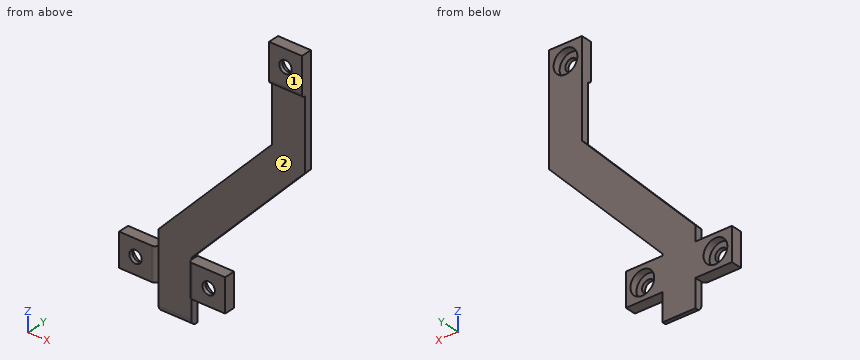
Autodesk Inventor part; units mm, degrees
ref_plane "YZ Plane" through (0, 0, 0) normal (1, 0, 0) x (0, 1, 0)
ref_plane "XZ Plane" through (0, 0, 0) normal (0, 1, 0) x (-1, 0, 0)
ref_plane "XY Plane" through (0, 0, 0) normal (0, 0, 1) x (1, 0, 0)
sketch "Sketch1" plane through (0, 0, 0) normal (0, 1, 0) x (-1, 0, 0)
  line L0 (0, 0) -> (-10, 0)
  line L1 (-10, 0) -> (-10, -51)
  line L2 (-10, -51) -> (0, -51)
  line L3 (0, -51) -> (0, 0)
  line L4 (0, 0) -> (-41, 0)
  line L5 (-41, 0) -> (-41, -10)
  line L6 (-41, -10) -> (0, -10)
  line L7 (0, -10) -> (0, 0)
  line L8 (-41, -10) -> (-31, -10)
  line L9 (-31, -10) -> (-31, 30)
  line L10 (-31, 30) -> (-41, 30)
  line L11 (-41, 30) -> (-41, -10)
  line L12 (-10, -51) -> (-10, -43)
  line L13 (-10, -43) -> (-20, -43)
  line L14 (-20, -43) -> (10, -43)
  line L15 (10, -43) -> (10, -33)
  line L16 (10, -33) -> (-20, -33)
  line L17 (-20, -33) -> (-20, -43)
  point P0 (0, -43)
  point P1 (0, -33)
  point P2 (-31, 0)
  point P3 (-10, -10)
  point P4 (-10, -33)
  dimension "d0" = 10
  dimension "d1" = 51
  dimension "d2" = 41
  dimension "d3" = 10
  dimension "d4" = 10
  dimension "d5" = 40
  dimension "d6" = 8
  dimension "d7" = 10
  dimension "d8" = 30
  dimension "d9" = 10
extrude "Extrusion1" add sketch "Sketch1" along normal blind 3
sketch "Sketch2" plane through (0, 3, 0) normal (0, 1, 0) x (1, 0, 0)
  line L0 (-10, 33) -> (0, 33)
  line L1 (0, 33) -> (0, 38)
  line L2 (0, 38) -> (-5, 38)
  circle A0 centre (-5, 38) radius 3.25
  line L3 (0, 38) -> (15, 38)
  circle A1 centre (15, 38) radius 3.25
  line L4 (41, -30) -> (41, 10)
  line L5 (41, -30) -> (41, -25)
  line L6 (41, -25) -> (41, -30)
  line L7 (41, -25) -> (36, -25)
  circle A2 centre (36, -25) radius 3.25
  circle A3 centre (-5, 38) radius 1.7
  circle A4 centre (15, 38) radius 1.7
  circle A5 centre (36, -25) radius 1.7
  point P0 (0, 0)
  dimension "d12" = 5
  dimension "d13" = 5
  dimension "d14" = 6.5
  dimension "d15" = 15
  dimension "d16" = 6.5
  dimension "d17" = 5
  dimension "d18" = 5
  dimension "d19" = 5
  dimension "d20" = 6.5
  dimension "d23" = 3.4
  dimension "d24" = 3.4
  dimension "d25" = 3.4
extrude "Extrusion3" cut sketch "Sketch2" against normal blind 2
extrude "Extrusion4" cut sketch "Sketch2" against normal blind 4 contours A3 | A4 | A5
sketch "Sketch3" plane through (0, 3, 0) normal (0, 1, 0) x (1, 0, 0)
  line L0 (0, 0) -> (0, 0.5)
  line L1 (0, 33) -> (0, 0)
  line L2 (0, 0.5) -> (31, 0.5)
  line L3 (31, 0.5) -> (31.5, 0.5)
  line L4 (31.5, 0.5) -> (31.5, -21.5)
  line L5 (31.5, -21.5) -> (40.5, -21.5)
  line L6 (31, -30) -> (41, -30)
  line L7 (40.5, -21.5) -> (40.5, 9.5)
  line L8 (41, -30) -> (41, 10)
  line L9 (40.5, 9.5) -> (9.5, 9.5)
  line L10 (9.5, 9.5) -> (9.5, 33.5)
  line L11 (9.5, 33.5) -> (19.5, 33.5)
  line L12 (20, 33) -> (20, 43)
  line L13 (19.5, 33.5) -> (19.5, 42.5)
  line L14 (19.5, 42.5) -> (9.5, 42.5)
  line L15 (9.5, 42.5) -> (9.5, 51)
  line L16 (10, 51) -> (0, 51)
  line L17 (10, 43) -> (10, 51)
  line L18 (9.5, 51) -> (10, 51)
  line L19 (10, 51) -> (10, 43)
  line L20 (20, 43) -> (10, 43)
  line L21 (20, 43) -> (10, 43)
  line L22 (10, 33) -> (20, 33)
  line L23 (20, 43) -> (20, 33)
  line L24 (20, 33) -> (10, 33)
  line L25 (10, 33) -> (10, 10)
  line L26 (41, 10) -> (10, 10)
  line L27 (10, 10) -> (41, 10)
  line L28 (41, 10) -> (41, -30)
  line L29 (31, 0) -> (31, -30)
  line L30 (41, -30) -> (31, -30)
  line L31 (31, -30) -> (31, 0)
  line L32 (31, 0) -> (0, 0)
  line L33 (0, 0.5) -> (0.5, 0.5)
  line L34 (0.5, 0.5) -> (0.5, 33.5)
  line L35 (9.5, 11.7035) -> (0.5, 11.7035)
  line L36 (5, 11.7035) -> (5, 17)
  line L37 (0.5, 9.5) -> (0.5, 33.5)
  line L38 (0.5, 33.5) -> (-9.5, 33.5)
  line L39 (-10, 33) -> (-10, 43)
  line L40 (-9.5, 33.5) -> (-9.5, 42.5)
  line L41 (-9.5, 42.5) -> (0.5, 42.5)
  line L42 (0.5, 42.5) -> (0.5, 51)
  line L43 (0, 51) -> (10, 51)
  line L44 (0, 43) -> (0, 51)
  line L45 (0.5, 51) -> (0, 51)
  line L46 (0, 51) -> (0, 43)
  line L47 (-10, 43) -> (0, 43)
  line L48 (-10, 43) -> (0, 43)
  line L49 (0, 33) -> (-10, 33)
  line L50 (-10, 43) -> (-10, 33)
  line L51 (-10, 33) -> (0, 33)
  line L52 (0, 33) -> (0, 10)
  line L53 (0, 0) -> (0.5, 0)
  line L54 (0.5, 0) -> (0.5, 33.5)
  line L55 (0.5, 33.5) -> (0, 33.5)
  line L56 (0, 33.5) -> (0, 0)
  dimension "d30" = 0.5
  dimension "d31" = 31
  dimension "d32" = 90
  dimension "d33" = 0.5
  dimension "d34" = 22
  dimension "d35" = 9
  dimension "d36" = 90
  dimension "d37" = 31
  dimension "d38" = 90
  dimension "d39" = 31
  dimension "d40" = 24
  dimension "d41" = 10
  dimension "d42" = 9
  dimension "d43" = 0.5
extrude "Extrusion5" cut sketch "Sketch3" against normal blind 4 contours L0 L2 L54 L32 | L1 L56 L38 L34 L2 | L54 L2 L3 L4 L5 L7 L9 L10 L11 L13 L14 L15 L16 L17 L20 L12 L22 L25 L26 L8 L6 L29 L32 | L49 L39 L47 L44 L16 L42 L41 L40 L38 L56
sketch "Sketch4" plane through (0, 3, 0) normal (0, 1, 0) x (1, 0, 0)
  line L0 (40.5, 9.5) -> (40.5, 38.6053)
  line L1 (9.5, 33.5) -> (46.5578, 33.5)
  line L2 (40.5, 33.5) -> (40.5, 0.5)
  line L3 (40.5, 9.5) -> (40.5, -21.5)
  line L4 (9.5, 9.5) -> (9.5, 33.5)
  line L5 (40.5, 0) -> (9.5, 33)
  line L6 (40.5, 0) -> (33.9404, -6.1621)
  line L7 (33.9404, -6.1621) -> (-17.219, 48.2979)
  line L8 (0.5, 33.5) -> (0.5, 0.5)
  line L9 (0.5, 33) -> (0.5, 28.5562)
  line L10 (19.5, 33.5) -> (9.5, 33.5)
  line L11 (9.5, 33) -> (0.5, 33)
  line L12 (9.5, 33.5) -> (9.5, 33)
  line L13 (9.5, 33.5) -> (9.5, 9.5)
  point P0 (0, 0)
  point P1 (0.5, 29.4357)
  point P2 (0.5, 33)
  dimension "d49" = 33
  dimension "d50" = 9
  dimension "d55" = 0.5
sketch "Sketch5" plane through (0, 3, 0) normal (0, 1, 0) x (1, 0, 0)
  line L0 (0.5, 33.5) -> (31.5, 33.5)
  line L1 (31.5, 33.5) -> (31.5, 9.5)
  line L2 (31.5, 0.5) -> (0.5, 0.5)
  line L3 (0.5, 0.5) -> (0.5, 33.5)
  line L4 (9.5, 9.5) -> (40.5, 9.5)
  line L5 (31.5, 0.5) -> (40.5, 0.5)
  line L6 (40.5, 0.5) -> (40.5, 9.5)
  line L7 (40.5, 9.5) -> (31.5, 9.5)
  point P0 (0, 0)
extrude "Extrusion6" cut sketch "Sketch5" against normal blind 4
extrude "Extrusion7" add sketch "Sketch4" against normal blind 3 contours L6 L7 L4 L5 | L4 L7 L8 L11
sketch "Sketch6" plane through (0, 3, 0) normal (0, 1, 0) x (1, 0, 0)
  line L0 (40.0303, 0.5) -> (9.5, 33)
  line L1 (33.4215, 7.5352) -> (47.7617, -7.7302)
  line L2 (47.7617, -7.7302) -> (49.311, 2.3426)
  line L3 (49.311, 2.3426) -> (33.4215, 7.5352)
  line L4 (9.5, 33) -> (0.5, 33)
  line L5 (-9.5, 33.5) -> (19.5, 33.5)
  line L6 (0.5, 33) -> (9.5, 33)
  line L7 (9.5, 33) -> (9.5, 33.5)
  line L8 (9.5, 33.5) -> (0.5, 33.5)
  line L9 (0.5, 33.5) -> (0.5, 33)
  point P0 (0, 0)
extrude "Extrusion8" add sketch "Sketch6" against normal blind 3 contours L4 L9 L5 L7
sketch "Sketch7" plane through (0, 3, 0) normal (0, 1, 0) x (1, 0, 0)
  line L0 (9.5, 33) -> (40.0303, 0.5)
  line L1 (37.6071, 3.0795) -> (42.3492, -1.9686)
  line L2 (42.3492, -1.9686) -> (43.0836, 1.6709)
  line L3 (43.0836, 1.6709) -> (37.6071, 3.0795)
  point P0 (0, 0)
  point P1 (40.0303, 0.5)
extrude "Extrusion9" cut sketch "Sketch7" against normal blind 3
sketch "Sketch10" plane through (0, 3, 0) normal (0, 1, 0) x (1, 0, 0)
  line L0 (40.5, -21.5) -> (31.5, -21.5)
  line L1 (31.5, -21.5) -> (31.5, -29.5)
  line L2 (31.5, -29.5) -> (40.5, -29.5)
  line L3 (40.5, -29.5) -> (40.5, -21.5)
  point P0 (0, 0)
  dimension "d60" = 9
  dimension "d61" = 8
extrude "Extrusion10" add sketch "Sketch10" against normal blind 3
sketch "Sketch11" plane through (0, 3, 0) normal (0, 1, 0) x (1, 0, 0)
  line L0 (31.5, -29.5) -> (40.5, -29.5)
  line L1 (36, -29.5) -> (36, -25)
  circle A0 centre (36, -25) radius 1.7
  point P0 (0, 0)
  dimension "d64" = 4.5
  dimension "d65" = 3.4
extrude "Extrusion11" cut sketch "Sketch11" against normal blind 3
sketch "Sketch12" plane through (0, 3, 0) normal (0, 1, 0) x (1, 0, 0)
  circle A0 centre (36, -25) radius 1.7
  circle A1 centre (36, -25) radius 3.25
  point P0 (0, 0)
  dimension "d68" = 6.5
extrude "Extrusion12" cut sketch "Sketch12" against normal blind 2
sketch "Sketch13" plane through (0, 3, 0) normal (0, 1, 0) x (1, 0, 0)
  line L0 (9.5, 51) -> (9.5, 42.5)
  line L1 (0.5, 42.5) -> (0.5, 51)
  line L2 (9.5, 51) -> (0.5, 51)
  line L3 (0.5, 51) -> (0.5, 48.5)
  line L4 (0.5, 48.5) -> (9.5, 48.5)
  line L5 (9.5, 48.5) -> (9.5, 51)
  point P0 (0, 0)
  point P1 (9.5, 48.5)
  dimension "d71" = 2.5
extrude "Extrusion13" cut sketch "Sketch13" against normal blind 3
sketch "Sketch14" plane through (0, 0, 0) normal (0, -1, 0) x (1, 0, 0)
  line L0 (9.5, -48.5) -> (0.5, -48.5)
  line L1 (9.5, -48.5) -> (0.5, -48.5)
  line L2 (0.5, -48.5) -> (0.5, -29.4357)
  line L3 (0.5, -29.4357) -> (9.5, -29.4357)
  line L4 (9.5, -29.4357) -> (9.5, -48.5)
  line L5 (-9.5, -33.5) -> (0.5, -33.5)
  line L6 (40.5, 29.5) -> (40.5, 0)
  line L7 (0.5, -33.5) -> (40.5, -33.5)
  line L8 (40.5, -33.5) -> (40.5, 19)
  line L9 (40.5, 19) -> (0.5, 19)
  line L10 (0.5, 19) -> (0.5, -33.5)
  point P0 (0, 0)
  point P1 (9.5, -33.5)
  point P2 (40.5, 0)
  dimension "d76" = 52.5
extrude "Extrusion14" cut sketch "Sketch14" against normal blind 1
fillet "Fillet4" radius 1 3 edges at (0.5, 0, -38) (9.5, 0, -38) (36, 0, 19)
sketch "Sketch15" plane through (0, 1, 0) normal (0, -1, 0) x (1, 0, 0)
  line L0 (9.5, -42.5) -> (9.5, -48.5)
  line L1 (9.5, -48.5) -> (0.5, -48.5)
  line L2 (0.5, -48.5) -> (0.5, -50)
  line L3 (0.5, -50) -> (9.5, -50)
  line L4 (9.5, -50) -> (9.5, -48.5)
  point P0 (0, 0)
  dimension "d81" = 9
  dimension "d82" = 1.5
extrude "Extrusion15" add sketch "Sketch15" against normal blind 2
fillet "Fillet6" radius 1.5 1 edges at (5, 1, -50)
properties part number "Cover_bottom_raceway_cover"
Work out the finished part from the listing and answer in its coordinate system (mm). Face numbers are marked on the shaded views. A direction names the side the tool comes from. Coordinates: 2 decimals unless noted, no trailing zeros. Loops run counter-clockwise (first coordinate to the right, second up) from the corner with the lowest first, then second, coordinate; pieces in that order, holes last. Notation, with made-up numbers: (19, 69) -> (60, 69) arc R9 cw to (60, 75) -> close; hole circle Ø6 at (73, 13.25). An arc over 180 degrees is marked (long way). Write each question's results on one line, items separated by ' | '. Start each with the question number.
1) Find section A-A on z = -38. Count the separate pieces of the cut face and the enclosed holes in it, then the cut area to 3 significant figures.
2) Find section D-D on x = 15. Determine the outline of the cut face in (y, z), then the cut area to 3 significant figures.
3) Find section B-B on x = -5. Determine the outline of the cut face in (y, z), then the cut area to 3 significant figures.
4) Consider line 1 along X through (y, z) = (0.2, 25); line 2 along X through (y, z) = (0.5, -38); line 3 along Z through (x, y) = (15, 1.6). Determine where each line is inside the solid, lowest interval first.
5) For the marked faces 1 and 2, determine the directions among +Z, -Z, +X, -X, +Y, -Y from which every point of the face is accessible in a straight line to the end or side of a thin tool.
6) Find section C-C on y = 0.5. Determine the outline of the cut face in (x, z), then the cut area to 3 significant figures.
7) Flat-ended cylindrical pins translate along their axes: P1, Ø3, axis at x = 11.5, z = -20.5, coming from the -Y side; P2, Ø2.5, axis at x = 36, z = 25, coming from the -Y side; P3, Ø0.9, axis at x = 16.5, y = 1.5, coming from the +Z side; P4, Ø1.6, axis at y = 2, z = -44.5, coming from the +X side. Find the tip coordinate at first contact, or state that the pin passes through.
Response values:
1) separate pieces: 3 | enclosed holes: 0 | area: 44.8 mm^2
2) outline: (0, -42.5) -> (3, -42.5) -> (3, -41.25) -> (1, -41.25) -> (1, -39.7) -> (0, -39.7) -> close; (0, -36.3) -> (1, -36.3) -> (1, -34.75) -> (3, -34.75) -> (3, -33.5) -> (0, -33.5) -> close; (1, -27.15) -> (3, -27.15) -> (3, -14) -> (1, -14) -> close | area: 36.9 mm^2
3) outline: (0, -42.5) -> (3, -42.5) -> (3, -41.25) -> (1, -41.25) -> (1, -39.7) -> (0, -39.7) -> close; (0, -36.3) -> (1, -36.3) -> (1, -34.75) -> (3, -34.75) -> (3, -33.5) -> (0, -33.5) -> close | area: 10.6 mm^2
4) line 1: x = 31.5 to 34.3, 37.7 to 40.5 | line 2: x = -9.5 to -6.7, -3.3 to 0.37, 9.63 to 13.3, 16.7 to 19.5 | line 3: z = -42.5 to -41.25, -34.75 to -33.5, -27.15 to -14
5) face 1: +Z, -Z, +X, -X, -Y | face 2: -Y
6) outline: (-9.5, -42.5) -> (0.37, -42.5) -> (0.37, -33.5) -> (-9.5, -33.5) -> close; (9.63, -42.5) -> (19.5, -42.5) -> (19.5, -33.5) -> (9.63, -33.5) -> close; (31.5, 19.13) -> (40.5, 19.13) -> (40.5, 29.5) -> (31.5, 29.5) -> close; hole circle Ø3.4 at (-5, -38); hole circle Ø3.4 at (15, -38); hole circle Ø3.4 at (36, 25) | area: 244 mm^2
7) P1: stops at y = 1 | P2: passes through | P3: stops at z = -11.92 | P4: stops at x = 9.5
